For this review, take the finished solid that the model builds, in its own axes (mm). Face numbers are marked on the shaded views. A direction names the side the tool comes from. Coordinates: 2 decimals unless noted, no trailing zeros. Order: outer loops, then holes, each group sorted by start corner. A loop starts at its lowest first (then second) coordinate and runs counter-clockwise, first axis right, second up. Notation, with made-up numbers: M 61,-2 L 83,-2 A17 ccw 83,4 Z; hole C -5.5,77 d4. An arc over 180 degrees is marked long. Use one line per item in the form item = value. Start each with the question number.
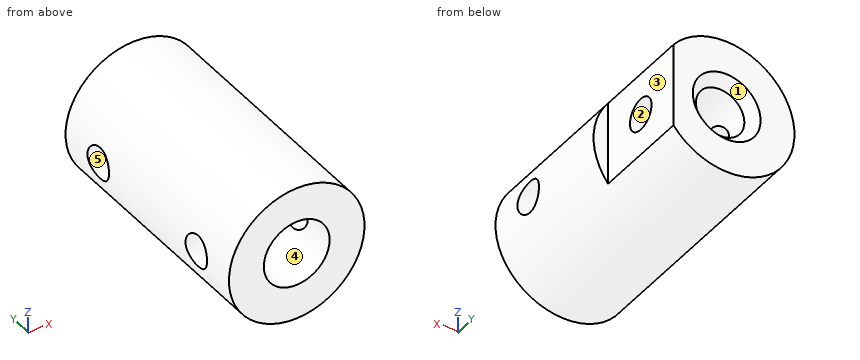
```python
from build123d import *

# Parameters (mm, degrees)
SKETCH1_W               = 4.5
SKETCH1_H               = 25
CUT_EXTRUDE1_DEPTH      = 27.888659319
CUT_EXTRUDE1_DEPTH_BACK = 27.888659319
SKETCH2_W               = 1.5
SKETCH2_H               = 10
CHAMFER1_SIZE           = 1
M8_TAPPED_HOLE1_D       = 6.8
M8_TAPPED_HOLE1_DEPTH   = 16
M8_TAPPED_HOLE1_TIP     = 2.042926105
M4_TAPPED_HOLE1_D       = 3.3


with BuildPart() as part:
    # Sketch1 → Revolve1 (revolve)
    with BuildSketch(Plane.XY, mode=Mode.PRIVATE) as revolve1_sk:
        with Locations((-4.75, 12.5)):
            Rectangle(SKETCH1_W, SKETCH1_H)
    revolve(revolve1_sk.sketch.rotate(Axis((0, 0, 0), (0, 1, 0)), 270), axis=Axis((0, 0, 0), (0, 1, 0)))

    # Sketch2 → Cut-Extrude1 (cut, two sides: drawn at the far end of the back side and taken through both)
    with BuildSketch(Plane.XY.offset(-CUT_EXTRUDE1_DEPTH_BACK)):
        with Locations((6.25, 20)):
            Rectangle(SKETCH2_W, SKETCH2_H)
    extrude(amount=CUT_EXTRUDE1_DEPTH + CUT_EXTRUDE1_DEPTH_BACK, mode=Mode.SUBTRACT)

    # Chamfer1
    chamfer1_edges = [part.edges().sort_by_distance(p)[0] for p in [
        (0, 25, 2.5),
    ]]
    chamfer(chamfer1_edges, length=CHAMFER1_SIZE)

    # M8 Tapped Hole1
    with Locations(Plane(origin=(0, 0, 0), x_dir=(-1, 0, 0), z_dir=(0, -1, 0))):
        with Locations((0, 0)):
            Hole(M8_TAPPED_HOLE1_D / 2, depth=M8_TAPPED_HOLE1_DEPTH)
            with Locations((0, 0, -(M8_TAPPED_HOLE1_DEPTH + M8_TAPPED_HOLE1_TIP / 2))):  # 118° drill point
                Cone(0, M8_TAPPED_HOLE1_D / 2, M8_TAPPED_HOLE1_TIP, mode=Mode.SUBTRACT)

    # M4 Tapped Hole1 (through all)
    with Locations(Plane(origin=(7, 0, 0), x_dir=(0, 0, -1), z_dir=(1, 0, 0))):
        with Locations((0, 20), (0, 5)):
            Hole(M4_TAPPED_HOLE1_D / 2)


solid = part.part
```
1. Tool access review of the marked faces 4 and 5: name each direction out of +Z, -Z, +X, -X, +Y, -Y from which nothing blocks a thin tool from reaching the whole face with its end or side.
2. The part is to be moulded in two halves that separate along X. For the marked faces 1, 2 and 3, say which applies: pulls with the +X half, pulls with the -X half, needs draft (parallel to the pull), parting line crosses it, or undercut.
3. For pin 1 Ø2 at (x, y) = (1.5, 13.5) entering from +Z; pin 2 Ø0.5 at (x, z) = (6.5, -2) entering from +Y; pin 3 Ø7 at (y, z) = (22, 0) entering from +X; pin 4 Ø2.5 at (y, z) = (20, 0) entering from -X, all flat-tipped, find the tip position at first contact; note any pin that passes through.
4. Consider section A-A, the plane z = 0. Give the number of separate pieces and of enclosed holes in the cut face, plus the area to 3 significant figures.
5. Consider section B-B, the plane x = 0. Write out the cut boundary in (y, z).
6. Consider section C-C, the plane y = 5. Write out the cut boundary in (x, z).
7. Consider section D-D, the plane y = 18. Write out the cut boundary in (x, z).
8. To check wall thickness, follow line 1 (Y direction, x = -4.45, z = 0); line 2 (Z direction, x = -5.5, y = 20); line 3 (Y direction, x = -5, z = 1.25). State the ranges of each line that lie inside material, in increasing order.
Answers follow:
q1.face_4 = -Y
q1.face_5 = +X, -X
q2.face_1 = undercut
q2.face_2 = needs draft
q2.face_3 = pulls with the +X half
q3.pin_1 = 6.98
q3.pin_2 = 15
q3.pin_3 = 5.5
q3.pin_4 = through
q4.separate_pieces = 6
q4.enclosed_holes = 0
q4.area = 131 mm²
q5.outline = M 0,-7 L 25,-7 L 25,-3.5 L 24,-2.5 L 16.54,-2.5 L 16,-3.4 L 0,-3.4 Z; M 0,3.4 L 16,3.4 L 16.54,2.5 L 24,2.5 L 25,3.5 L 25,7 L 0,7 Z
q6.outline = M -6.8,-1.65 A7 ccw 6.8,-1.65 L 2.97,-1.65 A3.4 cw -2.97,-1.65 Z; M -6.8,1.65 L -2.97,1.65 A3.4 cw 2.97,1.65 L 6.8,1.65 A7 ccw Z
q7.outline = M 5.5,-4.33 L 5.5,4.33 A7 ccw long Z; hole C 0,0 d5
q8.line_1 = 0 to 3.35, 6.65 to 18.35, 21.65 to 25
q8.line_2 = -4.33 to -1.65, 1.65 to 4.33
q8.line_3 = 0 to 3.92, 6.08 to 18.92, 21.08 to 25
